Source: CAD feature listing. Evaluate the final solid. Frame: model axes, mm. A direction names the side the tool comes from. Give positions to 0.01 mm unless a question says otherwise; leave off trailing zeros. Order: outer loops, then holes, each group sorted by start corner. A loop starts at its lowest first (then second) coordinate and runs counter-clockwise, first axis right, second up. Notation, with made-up numbers: (8.5, -6.75) - (39.5, -6.75) arc R28 cw to (39.5, 29.25) - close; hole circle Ø8 at (-20.5, -19). An arc over 180 degrees is marked (long way). Answer as CSV lines item,"result".
```python
from build123d import *

# Parameters (mm, degrees)
SKETCH4_R          = 1.25
CUT_EXTRUDE1_DEPTH = 5


with BuildPart() as part:
    # Sketch1 → Revolve1 (revolve)
    with BuildSketch(Plane.XY, mode=Mode.PRIVATE) as revolve1_sk:
        Polygon((0, 0), (73.3, 0), (73.3, 3), (61.3, 3), (61.3, 2.5), (60.5, 2.5), (60.5, 3), (60, 3), (60, 5), (6.1, 5), (6.1, 3), (5.6, 3), (5.6, 2.5), (4.8, 2.5), (4.8, 3), (0, 3), align=None)
    revolve(revolve1_sk.sketch.rotate(Axis((0, 0, 0), (1, 0, 0)), 180), axis=Axis((0, 0, 0), (1, 0, 0)))

    # Sketch4 → Cut-Extrude1 (cut, symmetric)
    with BuildSketch(Plane(origin=(0, 0, 0), x_dir=(-1, 0, 0), z_dir=(0, 0, -1))):
        with Locations((-71.52, 0)):
            Circle(SKETCH4_R)
    extrude(amount=CUT_EXTRUDE1_DEPTH, both=True, mode=Mode.SUBTRACT)


solid = part.part
```
(1) Access query for faces 1 (the flat face through (6.1, -3.3, -0.1)), 2 (the cylindrical face through (5.2, 2.5, -0.1)), 3 (the cylindrical face through (33, 5, 0)), 4 (the flat face through (73.3, 0, 0)), 5 (the cylindrical face through (67.22, -2.86, -0.9)). Directions: +Z, -Z, +X, -X, +Y, -Y. A direction counts if a zero-diameter tool reaches every point of the face in a straight line with its end or side. Return the directions, or none.
Completed:
face 1,"-X"
face 2,"none"
face 3,"+X, -X"
face 4,"+Z, -Z, +X, +Y, -Y"
face 5,"+X"
(2) Cut plane C-C (x = 59). Return loops of the section in (y, z), then the cut area to 3 significant figures.
Completed:
outline,"circle Ø10 at (0, 0)"
area,"78.5 mm²"
(3) Mould query, pull axis X, two halves, no side actions, for faces 6 (the flat face through (5.6, 2, -2)), 7 (the cylindrical face through (60.9, 2.5, -0.1)), 8 (the flat face through (0, 0, 0)), 9 (the cylindrical face through (2.37, -2.86, -0.9)). Classes: released by +X, released by -X, zero draft, split by the parting line, or undercut.
Completed:
face 6,"undercut"
face 7,"undercut"
face 8,"released by -X"
face 9,"zero draft"
(4) Cut plane D-D (x = 71.52). Return loops of the section in (y, z), then the cut area to 3 significant figures.
Completed:
outline,"(-1.25, -2.73) - (-1.25, 2.73) arc R3 ccw to start; (1.25, -2.73) arc R3 ccw to (1.25, 2.73) - close"
area,"13.7 mm²"
(5) Contact query for flat-ended pins moving along their axis: pin 1 (3 mm diameter, centred on y = 1.5, z = 0, fed in from -X); pin 2 (3 mm diameter, centred on x = 71.52, y = 0, fed in from +Z); pin 3 (1.5 mm diameter, centred on y = 1, z = -4, fed in from +X); pin 4 (5 mm diameter, centred on x = 58.5, y = -3.5, fed in from +Z). Output: stop coordinate, or through.
Completed:
pin 1,"x = 0"
pin 2,"z = 3"
pin 3,"x = 60"
pin 4,"z = 4.9"
(6) Ray query, line 1 (X direction, y = 0, z = -0.25); line 2 (X direction, y = -2.5, z = 1.5); line 3 (X direction, y = 3.25, z = 3.25). Return the intervals inside material, ascending. Write a range as from..to.
Completed:
line 1,"0..70.27, 72.77..73.3"
line 2,"0..4.8, 5.6..60.5, 61.3..73.3"
line 3,"6.1..60"
